from build123d import *

# Parameters (mm, degrees)
SKETCH1_W               = 24
SKETCH1_H               = 15.6
SKETCH2_W               = 193.8
SKETCH2_H               = 31.1
CUT_EXTRUDE1_DEPTH      = 44.6
CUT_EXTRUDE1_DEPTH_BACK = 44.6
HOLE1_D                 = 12.5
HOLE1_DEPTH             = 24.9


with BuildPart() as part:
    # Sketch1 → Revolve2 (revolve)
    with BuildSketch(Plane.XY):
        Polygon((0, 20), (0, 0), (341.8, 0), (341.8, 28), (118.2, 28), (94.2, 28), (28.9, 28), (28.9, 20), align=None)
        with Locations((106.2, 35.8)):
            Rectangle(SKETCH1_W, SKETCH1_H)
    revolve(axis=Axis((341.8, 0, 0), (-1, 0, 0)))

    # Sketch2 → Cut-Extrude1 (cut, two sides)
    with BuildSketch(Plane.XY) as cut_extrude1_sk:
        with Locations((229.8, 12.45)):
            Rectangle(SKETCH2_W, SKETCH2_H)
    extrude(amount=CUT_EXTRUDE1_DEPTH, mode=Mode.SUBTRACT)
    extrude(cut_extrude1_sk.sketch, amount=-CUT_EXTRUDE1_DEPTH_BACK, mode=Mode.SUBTRACT)

    # Hole1
    with Locations(Plane(origin=(0, -3.1, 0), x_dir=(1, 0, 0), z_dir=(0, 1, 0))):
        with Locations((179.8, 0), (279.8, 0)):
            Hole(HOLE1_D / 2, depth=HOLE1_DEPTH)


solid = part.part
The listing builds one solid part. Answer for the finished solid, in the listing's coordinates (mm). A direction names the side the tool comes from. Round coordinates to 2 decimals unless told otherwise and drop trailing zeros. Order: outer loops, then holes, each group sorted by start corner. A loop starts at its lowest first (then second) coordinate and runs counter-clockwise, first axis right, second up. Notation, with made-up numbers: (-22, 56.5) - (11, 56.5) arc R21 ccw to (11, 68.5) - close; hole circle Ø6 at (52.5, -1). An arc over 180 degrees is marked (long way). Write item = value, one per line. Start each with the question number.
1) For faces 1 (the flat face through (28.9, -7, -19)), 2 (the cylindrical face through (228.435, -27.973, -1.231)), 3 (the flat face through (132.9, 9, 0)), determine the directions among +Z, -Z, +X, -X, +Y, -Y from which every point of the face is accessible in a straight line to the end or side of a thin tool.
2) Given pin 1 (4 mm diameter, centred on y = 15.5, z = -30, fed in from -X); pin 2 (1 mm diameter, centred on y = 22, z = 31, fed in from +X); pin 3 (5 mm diameter, centred on x = 130.5, y = -24, fed in from -Z), each flat-ended and moving along its own axis, determine where each tip first touches the part or whether it passes through.
3) Section A-A, the plane z = 0 is taken. Write down the section's boundary in (x, y).
4) Straight lines are drawn through the part: L1, parallel to X at y = -18.5, z = 22.5; L2, parallel to X at y = -24, z = -7.5; L3, parallel to Z at x = 279.8, y = -22.5. For each, find the intervals that lie inside material, in ascending order.
5) For a pull along Z with two mould halves and no side action, classify faces 4 (the flat face through (118.2, 0.6, 28.5)), 5 (the cylindrical face through (186.044, -15.725, -0.275)), 6 (the cylindrical face through (61.093, 25.865, 10.724)) as released by +Z, released by -Z, zero draft, split by the parting line, or undercut.
6) Section B-B, the plane y = 0 is taken. Write down the section's boundary in (x, z).
7) Section D-D, the plane x = 24 is taken. Write down the section's boundary in (y, z), plus the area to 3 significant figures.
8) Section C-C, the plane x = 179.8 is taken. Write down the section's boundary in (y, z).
Results list:
q1.face_1 = -X
q1.face_2 = +X
q1.face_3 = +Z, -Z, +Y
q2.pin_1 = 94.2
q2.pin_2 = 118.2
q2.pin_3 = -17.94
q3.outline = (0, -20) - (28.9, -20) - (28.9, -28) - (94.2, -28) - (94.2, -43.6) - (118.2, -43.6) - (118.2, -28) - (173.55, -28) - (173.55, -3.1) - (132.9, -3.1) - (132.9, 28) - (118.2, 28) - (118.2, 43.6) - (94.2, 43.6) - (94.2, 28) - (28.9, 28) - (28.9, 20) - (0, 20) - close; (186.05, -28) - (273.55, -28) - (273.55, -3.1) - (186.05, -3.1) - close; (286.05, -28) - (341.8, -28) - (341.8, 28) - (326.7, 28) - (326.7, -3.1) - (286.05, -3.1) - close
q4.L1 = 94.2 to 118.2
q4.L2 = 28.9 to 341.8
q4.L3 = -16.67 to -6.25, 6.25 to 16.67
q5.face_4 = zero draft
q5.face_5 = undercut
q5.face_6 = split by the parting line
q6.outline = (0, -20) - (28.9, -20) - (28.9, -28) - (94.2, -28) - (94.2, -43.6) - (118.2, -43.6) - (118.2, -28) - (132.9, -28) - (132.9, 28) - (118.2, 28) - (118.2, 43.6) - (94.2, 43.6) - (94.2, 28) - (28.9, 28) - (28.9, 20) - (0, 20) - close; (326.7, -28) - (341.8, -28) - (341.8, 28) - (326.7, 28) - close
q7.outline = circle Ø40 at (0, 0)
q7.area = 1,260 mm^2
q8.outline = (-27.29, -6.25) arc R28 ccw to (-3.1, -27.83) - (-3.1, -6.25) - close; (-27.29, 6.25) - (-3.1, 6.25) - (-3.1, 27.83) arc R28 ccw to start
